from build123d import *

# Parameters (mm, degrees)
SKETCH1_R           = 62.5
SKETCH1_R_2         = 57.5
BOSS_EXTRUDE1_DEPTH = 10
SKETCH2_R           = 62.5
BOSS_EXTRUDE2_DEPTH = 22
SKETCH3_R           = 2.5
CUT_EXTRUDE1_DEPTH  = 92.08512502
CUT_EXTRUDE2_DEPTH  = 18
SKETCH5_R           = 6
SKETCH5_R_2         = 2.5
BOSS_EXTRUDE3_DEPTH = 8
SKETCH6_R           = 1.5
CUT_EXTRUDE3_DEPTH  = 98.01803956
SKETCH7_R           = 2.5
CUT_EXTRUDE4_DEPTH  = 98.018039601
CIRPATTERN1_COUNT   = 3
SKETCH8_R           = 2
CUT_EXTRUDE5_DEPTH  = 93.717312465


with BuildPart() as part:
    # Sketch1 → Boss-Extrude1 (new body)
    with BuildSketch(Plane.XY):
        Circle(SKETCH1_R)
        Circle(SKETCH1_R_2, mode=Mode.SUBTRACT)
    extrude(amount=BOSS_EXTRUDE1_DEPTH)

    # Sketch2 → Boss-Extrude2 (add)
    with BuildSketch(Plane.XY.offset(10)):
        Circle(SKETCH2_R)
    extrude(amount=BOSS_EXTRUDE2_DEPTH)

    # Sketch3 → Cut-Extrude1 (cut, through all)
    with BuildSketch(Plane(origin=(0, 0, 10), x_dir=(-1, 0, 0), z_dir=(0, 0, -1))):
        Circle(SKETCH3_R)
    extrude(amount=-CUT_EXTRUDE1_DEPTH, mode=Mode.SUBTRACT)

    # Sketch4 → Cut-Extrude2 (cut)
    with BuildSketch(Plane(origin=(0, 0, 10), x_dir=(-1, 0, 0), z_dir=(0, 0, -1))):
        with BuildLine():
            Line((0, 16), (74.659744803, 16))
            Line((74.659744803, 16), (74.659744803, -16))
            Line((74.659744803, -16), (0, -16))
            ThreePointArc((0, -16), (-16, 0), (0, 16))
        make_face()
    extrude(amount=-CUT_EXTRUDE2_DEPTH, mode=Mode.SUBTRACT)

    # Sketch5 → Boss-Extrude3 (add)
    with BuildSketch(Plane.XY.offset(32)):
        Circle(SKETCH5_R)
        with Locations(Location((0, 0, 0), (0, 0, 180))):
            Circle(SKETCH5_R_2, mode=Mode.SUBTRACT)
    extrude(amount=BOSS_EXTRUDE3_DEPTH)

    # Sketch6 → Cut-Extrude3 (cut, through all)
    with BuildSketch(Plane(origin=(0, 0, 0), x_dir=(1, 0, 0), z_dir=(0, 1, 0))):
        with Locations(Location((0, -37, 0), (0, 0, 270))):
            Circle(SKETCH6_R)
    extrude(amount=-CUT_EXTRUDE3_DEPTH, mode=Mode.SUBTRACT)

    # Sketch7 → Cut-Extrude4 (cut, through all)
    with BuildSketch(Plane(origin=(0, 0, 0), x_dir=(1, 0, 0), z_dir=(0, 1, 0))):
        with Locations(Location((0, -6, 0), (0, 0, 270))):
            Circle(SKETCH7_R)
    cut_extrude4 = extrude(amount=-CUT_EXTRUDE4_DEPTH, mode=Mode.SUBTRACT)

    # CirPattern1: Cut-Extrude4 ×3 about axis
    cirpattern1_axis = Axis((0, 0, 0), (0, 0, 1))
    for i in range(1, CIRPATTERN1_COUNT):
        add(cut_extrude4.rotate(cirpattern1_axis, i * 360 / CIRPATTERN1_COUNT), mode=Mode.SUBTRACT)

    # Sketch8 → Cut-Extrude5 (cut, through all)
    with BuildSketch(Plane(origin=(0, 0, 28), x_dir=(-1, 0, 0), z_dir=(0, 0, -1))):
        with Locations(Location((40, 10, 0), (0, 0, 90))):
            Circle(SKETCH8_R)
        with Locations(Location((40, -10, 0), (0, 0, 90))):
            Circle(SKETCH8_R)
    extrude(amount=-CUT_EXTRUDE5_DEPTH, mode=Mode.SUBTRACT)


solid = part.part
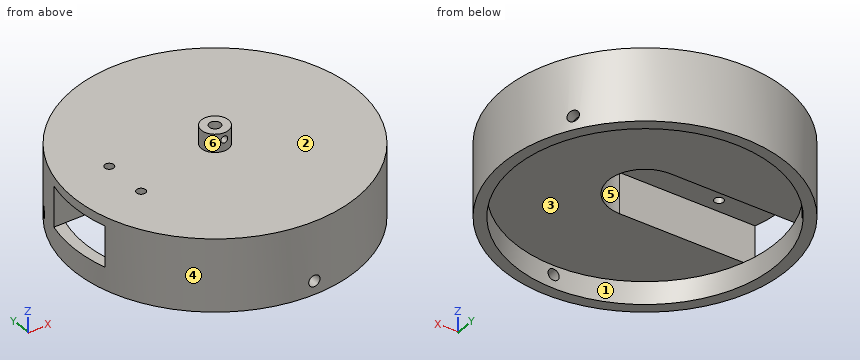
The model under review builds one solid part; all positions refer to its coordinate system, in mm. Face numbers are marked on the shaded views. A direction names the side the tool comes from. Coordinates: 2 decimals unless noted, no trailing zeros. Loops run counter-clockwise (first coordinate to the right, second up) from the corner with the lowest first, then second, coordinate; pieces in that order, holes last. Notation, with made-up numbers: M 45.5,59.25 L 82.5,59.25 A24 ccw 82.5,92.25 Z; hole C -37,86 d4. An arc over 180 degrees is marked long. Put each result on its own line as item: value. Start each with the question number.
Q1. Add section A-A (z = 6). Write out the cut boundary in (x, y), and give its area (3 significant figures).
Q2. The part is to be moulded in two halves that separate along Y. For the marked faces 1, 2, 3 and 4, say which applies: +Y half, -Y half, draft (parallel to the pull), parting line (faces both ways), or undercut.
Q3. Clearance check with flat-ended pins moving along their axes: pin 1 (1.5 mm diameter, centred on y = -7.5, z = 9.5, fed in from +X); pin 2 (3 mm diameter, centred on x = 28.5, z = 13.5, fed in from -Y); pin 3 (8 mm diameter, centred on x = -60.5, y = -6, fed in from +Z). State where each tip first meets the part, or that it passes through.
Q4. Wall thickness on line 1 (X direction, y = 0, z = 5); line 2 (Y direction, x = 0, z = 33); line 3 (Z direction, x = 0, y = -59): over which ranges is each line inside the solid? List them lowest first.
Q5. Add section C-C (y = -35). Write out the cut boundary in (x, z), and give its area (3 significant figures).
Q6. For the marked faces 5 and 6, list the 3-axis set-ups (+Z, -Z, +X, -X, +Y, -Y) from which the entire face can be reached by the end or side of a thin tool; tool diameter is ignored.
Q7. Add section B-B (x = -40). Write out the cut boundary in (y, z), and give its area (3 significant figures).
Q8. Add section D-D (y = -10). Write out the cut boundary in (x, z), and give its area (3 significant figures).
Answers:
1. outline: M -55.33,29.06 A62.5 ccw -2.5,-62.45 L -2.5,-57.45 A57.5 cw -51,26.56 Z; M -52.83,33.39 L -48.5,30.89 A57.5 cw 48.5,30.89 L 52.83,33.39 A62.5 ccw Z; M 2.5,-62.45 A62.5 ccw 55.33,29.06 L 51,26.56 A57.5 cw 2.5,-57.45 Z
1. area: 1,810 mm^2
2. face 1: undercut
2. face 2: draft
2. face 3: undercut
2. face 4: parting line
3. pin 1: stops at x = 62.13
3. pin 2: stops at y = -56.37
3. pin 3: stops at z = 32
4. line 1: x = -62.5 to -57.5, 57.5 to 62.5
4. line 2: y = -6 to -2.5, 2.5 to 6
4. line 3: z = 0 to 3.5, 8.5 to 32
5. outline: M -51.78,0 L -45.62,0 L -45.62,10 L 45.62,10 L 45.62,0 L 51.78,0 L 51.78,32 L -51.78,32 Z
5. area: 2,400 mm^2
6. face 5: -Z, -X
6. face 6: +Z
7. outline: M -48.02,0 L -41.31,0 L -41.31,10 L -16,10 L -16,28 L -12,28 L -12,32 L -48.02,32 Z; M -8,28 L 8,28 L 8,32 L -8,32 Z; M 12,28 L 16,28 L 16,10 L 41.31,10 L 41.31,0 L 48.02,0 L 48.02,32 L 12,32 Z
7. area: 1,640 mm^2
8. outline: M -61.69,0 L -56.62,0 L -56.62,10 L -61.69,10 Z; M -61.69,28 L -42,28 L -42,32 L -61.69,32 Z; M -38,28 L 12.49,28 L 12.49,10 L 56.62,10 L 56.62,0 L 61.69,0 L 61.69,32 L -38,32 Z
8. area: 1,460 mm^2
